For this review, take the finished solid that the model builds, in its own axes (mm). A direction names the side the tool comes from. Coordinates: 2 decimals unless noted, no trailing zeros. Write each loop counter-clockwise with the first axis right and the second up, starting at its lowest first coordinate (ties: lowest second). Pieces come first, ordered by that corner, then holes. Notation, with made-up numbers: M 42,29.5 L 58,29.5 A25 cw 58,51.5 Z; hole C 46.25,-7 d7. An arc over 180 degrees is marked long. One line per question, with ' | ' between items.
from build123d import *

# Parameters (mm, degrees)
SM_BASE_FLANGE_1_DEPTH = 110
M3X0_5_1_D             = 2.5
M3X0_5_1_DEPTH         = 8.5
M3X0_5_1_TIP           = 0.751075774
CHAMFER_1_SIZE         = 5
CUT_EXTRUDE_1_REACH    = 192.263
SKETCH_8_R             = 1.65


# Sheet-metal steps are written as plain solids
with BuildPart() as part:
    # Sketch 1 → 基材-凸緣1 (new body)
    with BuildSketch(Plane.XY):
        with BuildLine():
            Line((-40, 0), (-0.7366, 0))
            ThreePointArc((-0.7366, 0), (-0.215745145, 0.215745145), (0, 0.7366))
            Line((0, 0.7366), (0, 150))
            Line((0, 150), (3, 150))
            Line((3, 150), (3, 0.7366))
            ThreePointArc((3, 0.7366), (1.905575199, -1.905575199), (-0.7366, -3))
            Line((-0.7366, -3), (-40, -3))
            Line((-40, -3), (-40, 0))
        make_face()
    extrude(amount=SM_BASE_FLANGE_1_DEPTH)

    # M3x0.5 螺紋孔1
    with Locations(Plane.ZY):
        with Locations((10, 140.3683), (100, 140.3683), (100, 10.3683), (10, 10.3683)):
            Hole(M3X0_5_1_D / 2, depth=M3X0_5_1_DEPTH)
            with Locations((0, 0, -(M3X0_5_1_DEPTH + M3X0_5_1_TIP / 2))):  # 118° drill point
                Cone(0, M3X0_5_1_D / 2, M3X0_5_1_TIP, mode=Mode.SUBTRACT)

    # 導角1
    chamfer_1_edges = [part.edges().sort_by_distance(p)[0] for p in [
        (-40, -1.5, 110),
        (-40, -1.5, 0),
        (1.5, 150, 110),
        (1.5, 150, 0),
    ]]
    chamfer(chamfer_1_edges, length=CHAMFER_1_SIZE)

    # 草圖8 → 除料-伸長1 (cut, up to next)
    with BuildSketch(Plane(origin=(0, 0, 0), x_dir=(1, 0, 0), z_dir=(0, 1, 0)), mode=Mode.PRIVATE) as cut_extrude_1_sk1:
        with Locations(Location((-10, -20, 0), (0, 0, 270))):
            Circle(SKETCH_8_R)
    cut_extrude_1_tool1 = extrude(cut_extrude_1_sk1.sketch, amount=-CUT_EXTRUDE_1_REACH, mode=Mode.PRIVATE) & part.part
    # 草圖8 → 除料-伸長1 (cut, up to next)
    with BuildSketch(Plane(origin=(0, 0, 0), x_dir=(1, 0, 0), z_dir=(0, 1, 0)), mode=Mode.PRIVATE) as cut_extrude_1_sk2:
        with Locations(Location((-10, -90, 0), (0, 0, 270))):
            Circle(SKETCH_8_R)
    cut_extrude_1_tool2 = extrude(cut_extrude_1_sk2.sketch, amount=-CUT_EXTRUDE_1_REACH, mode=Mode.PRIVATE) & part.part
    # 草圖8 → 除料-伸長1 (cut, up to next)
    with BuildSketch(Plane(origin=(0, 0, 0), x_dir=(1, 0, 0), z_dir=(0, 1, 0)), mode=Mode.PRIVATE) as cut_extrude_1_sk3:
        with Locations(Location((-30, -90, 0), (0, 0, 270))):
            Circle(SKETCH_8_R)
    cut_extrude_1_tool3 = extrude(cut_extrude_1_sk3.sketch, amount=-CUT_EXTRUDE_1_REACH, mode=Mode.PRIVATE) & part.part
    # 草圖8 → 除料-伸長1 (cut, up to next)
    with BuildSketch(Plane(origin=(0, 0, 0), x_dir=(1, 0, 0), z_dir=(0, 1, 0)), mode=Mode.PRIVATE) as cut_extrude_1_sk4:
        with Locations(Location((-30, -20, 0), (0, 0, 270))):
            Circle(SKETCH_8_R)
    cut_extrude_1_tool4 = extrude(cut_extrude_1_sk4.sketch, amount=-CUT_EXTRUDE_1_REACH, mode=Mode.PRIVATE) & part.part
    add(cut_extrude_1_tool1.solids().sort_by_distance((-10, 0, 20))[0], mode=Mode.SUBTRACT)
    add(cut_extrude_1_tool2.solids().sort_by_distance((-10, 0, 90))[0], mode=Mode.SUBTRACT)
    add(cut_extrude_1_tool3.solids().sort_by_distance((-30, 0, 90))[0], mode=Mode.SUBTRACT)
    add(cut_extrude_1_tool4.solids().sort_by_distance((-30, 0, 20))[0], mode=Mode.SUBTRACT)


solid = part.part
1. Draft analysis for pull direction X (two halves, no side actions). For faces 3 (the flat face through (1, 150, 54)), 4 (the flat face through (3, 76, 54)), 5 (the cylindrical face through (-28.885, -1.479, 88.784)), state which applies: pulls with the +X half, pulls with the -X half, needs draft (parallel to the pull), parting line crosses it, or undercut.
Computed values:
face 3: needs draft | face 4: pulls with the +X half | face 5: undercut
2. Take a section at B-B on x = -30. State the section outline as (y, z) points, plus the area to 3 significant figures.
Computed values:
outline: M -3,0 L 0,0 L 0,18.35 L -3,18.35 Z; M -3,21.65 L 0,21.65 L 0,88.35 L -3,88.35 Z; M -3,91.65 L 0,91.65 L 0,110 L -3,110 Z | area: 310 mm2
3. Take a section at A-A on z = 90. State the section outline as (x, y) points, plus the area to 3 significant figures.
Computed values:
outline: M -40,-3 L -31.65,-3 L -31.65,0 L -40,0 Z; M -28.35,-3 L -11.65,-3 L -11.65,0 L -28.35,0 Z; M -8.35,-3 L -0.74,-3 A3.74 ccw 3,0.74 L 3,150 L 0,150 L 0,0.74 A0.74 cw -0.74,0 L -8.35,0 Z | area: 556 mm2
4. For line 1 along Y through (x, z) = (0.7, 100); line 2 along X through (y, z) = (-1.2, 90); line 3 along Y through (x, z) = (-18, 39), list the stretches that pass through material, from the lowest coordinate up.
Computed values:
line 1: y = -2.71 to 9.12, 11.62 to 139.12, 141.62 to 150 | line 2: x = -40 to -31.65, -28.35 to -11.65, -8.35 to 2.46 | line 3: y = -3 to 0
5. Clearance check with flat-ended pins moving along their axes: P1, Ø4, axis at y = 32, z = 83, coming from the -X side; P2, Ø4.5, axis at x = -30, z = 20, coming from the +Y side. State where each tip first meets the part, or that it passes through.
Computed values:
P1: stops at x = 0 | P2: stops at y = 0
6. Machinability: for faces 1 (the flat face through (0, 74, 54)), 2 (the flat face through (-37, -2, 2)), which of the approach directions +Z, -Z, +X, -X, +Y, -Y give a long, thin tool a straight path to every point of the face, cutting with its end or side? Answer none if there is none.
Computed values:
face 1: +Z, -Z, -X, +Y | face 2: -Z, -X, +Y, -Y
7. Take a section at C-C on z = 27.5. State the section outline as (x, y) points.
Computed values:
outline: M -40,-3 L -0.74,-3 A3.74 ccw 3,0.74 L 3,150 L 0,150 L 0,0.74 A0.74 cw -0.74,0 L -40,0 Z
8. Take a section at D-D on y = 125.5. State the section outline as (x, z) points, plus the area to 3 significant figures.
Computed values:
outline: M 0,0 L 3,0 L 3,110 L 0,110 Z | area: 330 mm2
